Can you work these out from the drawing? Everything is in mm from the part's minimum corner. Round coordinates to 2 decimals unless told otherwise and drop trailing zeros. Order: outer loops, then holes, each group sorted by start corner. A loop starts at its lowest first (then second) coordinate and runs counter-clockwise, first axis right, second up. Notation, with made-up numbers: (42, -28.75) -> (83, -28.75) arc R34 cw to (83, 9.25) -> close; hole circle Ø6 at (-26.75, 80.5). An arc over 180 degrees is marked (long way). One line per item, written item: value.
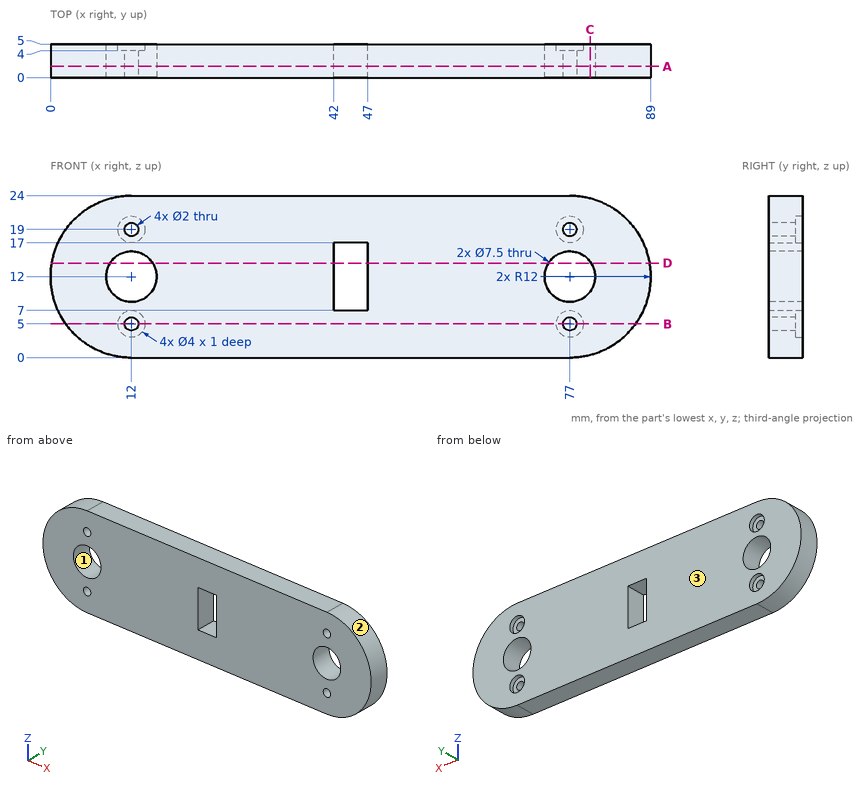
Q1. I want a section at C-C on x = 80. List the corners of the cut face in (y, z) for me, plus the area to 3 significant figures.
Answers below:
outline: (0, 0.38) -> (5, 0.38) -> (5, 9.75) -> (0, 9.75) -> close; (0, 14.25) -> (5, 14.25) -> (5, 23.62) -> (0, 23.62) -> close
area: 93.7 mm^2
Q2. We'd pull the mould along Z, two halves only. Please class the marked faces 1, 2 and 3: released by +Z, released by -Z, zero draft, split by the parting line, or undercut.
Answers below:
face 1: undercut
face 2: split by the parting line
face 3: zero draft
Q3. I want a section at A-A on y = 1.7. List the corners of the cut face in (x, z) for me, plus the area to 3 significant figures.
Answers below:
outline: (12, 0) -> (77, 0) arc R12 ccw to (77, 24) -> (12, 24) arc R12 ccw to start; hole circle Ø7.5 at (12, 12); hole circle Ø2 at (12, 5); hole circle Ø2 at (12, 19); hole (42, 7) -> (47, 7) -> (47, 17) -> (42, 17) -> close; hole circle Ø7.5 at (77, 12); hole circle Ø2 at (77, 5); hole circle Ø2 at (77, 19)
area: 1,860 mm^2
Q4. I want a section at B-B on z = 5. List the corners of the cut face in (x, y) for me.
Answers below:
outline: (2.25, 0) -> (11, 0) -> (11, 4) -> (10, 4) -> (10, 5) -> (2.25, 5) -> close; (13, 0) -> (76, 0) -> (76, 4) -> (75, 4) -> (75, 5) -> (14, 5) -> (14, 4) -> (13, 4) -> close; (78, 0) -> (86.75, 0) -> (86.75, 5) -> (79, 5) -> (79, 4) -> (78, 4) -> close
Q5. Please list where these lines run through material, in increasing order: line 1 along X through (y, z) = (2.7, 12); line 2 along Z through (x, y) = (77, 4.3); line 3 along Z through (x, y) = (12, 1.05).
Answers below:
line 1: 0 to 8.25, 15.75 to 42, 47 to 73.25, 80.75 to 89
line 2: 0 to 3, 7 to 8.25, 15.75 to 17, 21 to 24
line 3: 0 to 4, 6 to 8.25, 15.75 to 18, 20 to 24
Q6. I want a section at D-D on z = 14. List the corners of the cut face in (x, y) for me, plus the area to 3 significant figures.
Answers below:
outline: (0.17, 0) -> (8.83, 0) -> (8.83, 5) -> (0.17, 5) -> close; (15.17, 0) -> (42, 0) -> (42, 5) -> (15.17, 5) -> close; (47, 0) -> (73.83, 0) -> (73.83, 5) -> (47, 5) -> close; (80.17, 0) -> (88.83, 0) -> (88.83, 5) -> (80.17, 5) -> close
area: 355 mm^2
Q7. Will these pins go through, and if not, where does the flat tip stop? pin 1 Ø10 at (x, z) = (12, 12) entering from -Y; pin 2 Ø2.5 at (x, z) = (12, 5) entering from +Y; pin 3 Ø2 at (y, z) = (1, 19) entering from -X; pin 4 Ø1 at (y, z) = (2.5, 13) entering from +X.
Answers below:
pin 1: y = 0
pin 2: y = 4
pin 3: x = 1.61
pin 4: x = 88.99
